Source: CAD feature listing. Evaluate the final solid. Frame: model axes, mm. Face numbers are marked on the shaded views. Coordinates: 2 decimals unless noted, no trailing zeros. Order: outer loops, then holes, each group sorted by start corner. A loop starts at its lowest first (then second) coordinate and runs counter-clockwise, first axis right, second up. Notation, with made-up numbers: (-27.5, -30) -> (-2.5, -30) arc R19 ccw to (-2.5, -13) -> close; hole circle Ø11 at (-31, 16.5). An arc over 180 degrees is marked (long way). Write item = value, one per line. Start each with the question number.
Item 1: Section query D-D (y = 1). Output: boundary loops of the cut face in (x, z), then the cut area to 3 significant figures.
Item 2: Section query C-C (z = 0). Output: boundary loops of the cut face in (x, y) (3 decimals).
Item 3: Mould query, pull axis X, two halves, no side actions, for the marked faces 1 and 2. Classes: released by +X, released by -X, zero draft, split by the parting line, or undercut.
Item 4: Section query B-B (z = -17.5). Output: boundary loops of the cut face in (x, y) (1 decimal).
Item 5: Ray query, line 1 along Z through (x, y) = (0, 2.25); line 2 along Y through (x, z) = (-21, 1.5) (3 decimals); line 3 along X through (y, z) = (2, -19.05). Return the intervals inside material, ascending. Write a range as [from, to].
Item 6: Contact query for flat-ended pins moving along their axis: pin 1 (3 mm diameter, centred on y = 3, z = 8, fed in from +X); pin 2 (3.5 mm diameter, centred on x = 8.5, z = -1, fed in from +Y) (3 decimals); pin 3 (3 mm diameter, centred on y = 1.5, z = 10.5, fed in from +X). Output: stop coordinate, or through.
Item 7: Section query A-A (y = 5.75). Output: boundary loops of the cut face in (x, z) (3 decimals), then the cut area to 3 significant figures.
Autodesk Inventor part; units mm, degrees
ref_plane "YZ Plane" through (0, 0, 0) normal (1, 0, 0) x (0, 1, 0)
ref_plane "XZ Plane" through (0, 0, 0) normal (0, 1, 0) x (-1, 0, 0)
ref_plane "XY Plane" through (0, 0, 0) normal (0, 0, 1) x (1, 0, 0)
sketch "Sketch1" plane through (0, 0, 0) normal (0, 1, 0) x (-1, 0, 0)
  circle A0 centre (0, 0) radius 25.4
  circle A1 centre (0, -19.05) radius 2.159
  circle A2 centre (0, 19.05) radius 2.159
  line L0 (0, 19.05) -> (0, -19.05)
  dimension "d0" = 50.8
  dimension "d1" = 4.318
  dimension "d2" = 4.318
  dimension "d3" = 38.1
extrude "Extrusion1" add sketch "Sketch1" along normal blind 3.175
sketch "Sketch2" plane through (0, 3.175, 0) normal (0, 1, 0) x (1, 0, 0)
  arc A0 (0.2258, 3.4927) -> (0.2258, -3.4927) centre (0, 0) ccw
  arc A1 (15.6613, -2.4948) -> (15.6613, 2.4948) centre (15.5, 0) ccw
  line L0 (0.2258, 3.4927) -> (15.6613, 2.4948)
  line L1 (15.6613, -2.4948) -> (0.2258, -3.4927)
  line L2 (15.8661, 5.6632) -> (0.4306, 6.6611)
  arc A2 (0.4306, 6.6611) -> (0.4306, -6.6611) centre (0, 0) ccw
  line L3 (0.4306, -6.6611) -> (15.8661, -5.6632)
  arc A3 (15.8661, -5.6632) -> (15.8661, 5.6632) centre (15.5, 0) ccw
  dimension "d6" = 7
  dimension "d7" = 5
  dimension "d8" = 21.5
  dimension "d9" = 3.175
extrude "Extrusion2" add sketch "Sketch2" along normal blind 3.175
properties part number "Thingy"
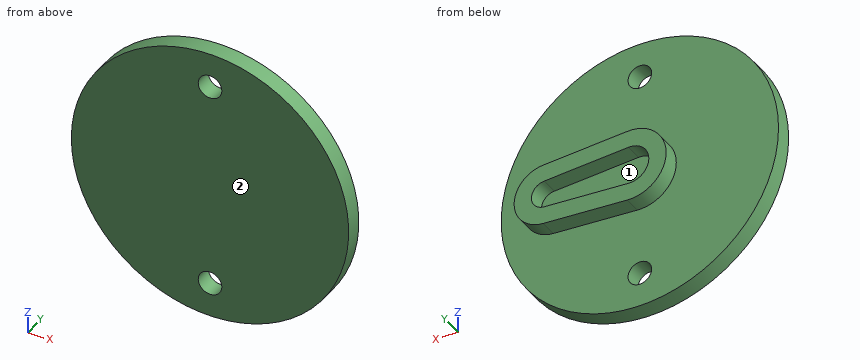
Computed:
q1.outline = circle Ø50.8 at (0, 0); hole circle Ø4.32 at (0, -19.05); hole circle Ø4.32 at (0, 19.05)
q1.area = 2,000 mm^2
q2.outline = (-25.4, 0) -> (25.4, 0) -> (25.4, 3.175) -> (21.175, 3.175) -> (21.175, 6.35) -> (18, 6.35) -> (18, 3.175) -> (-3.5, 3.175) -> (-3.5, 6.35) -> (-6.675, 6.35) -> (-6.675, 3.175) -> (-25.4, 3.175) -> close
q3.face_1 = undercut
q3.face_2 = zero draft
q4.outline = (-18.4, 0) -> (-1.5, 0) -> (-1.5, 3.2) -> (-18.4, 3.2) -> close; (1.5, 0) -> (18.4, 0) -> (18.4, 3.2) -> (1.5, 3.2) -> close
q5.line_1 = [-25.4, -21.21], [-16.89, 16.89], [21.21, 25.4]
q5.line_2 = [0, 3.175]
q5.line_3 = [-16.8, -2.16], [2.16, 16.8]
q6.pin_1 = 24.55
q6.pin_2 = 3.175
q6.pin_3 = 23.75
q7.outline = (0.431, -6.661) -> (15.866, -5.663) arc R5.675 ccw to (15.866, 5.663) -> (0.431, 6.661) arc R6.675 ccw (long way) to start; hole (0.226, -3.493) -> (15.661, -2.495) arc R2.5 ccw to (15.661, 2.495) -> (0.226, 3.493) arc R3.5 ccw (long way) to start
q7.area = 190 mm^2
